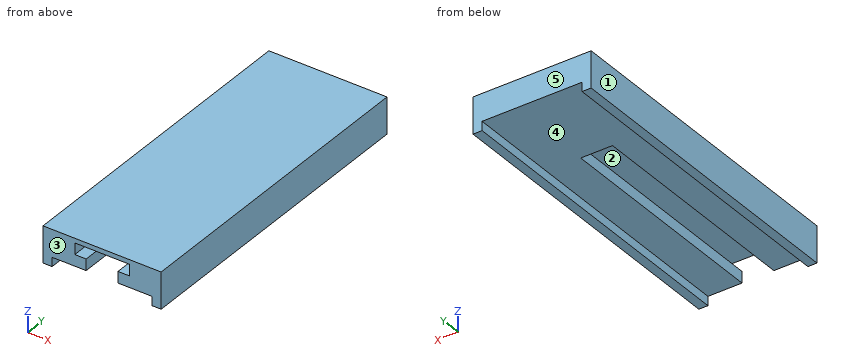
```python
from build123d import *

# Parameters (mm, degrees)
F1_DEPTH = 70
F3_DEPTH = 50


with BuildPart() as f1:
    # F0 (on Front) → F1 (new body)
    with BuildSketch(Plane.XZ):
        Polygon((-11, -6), (11, -6), (11, -8), (13, -8), (13, 0), (-13, 0), (-13, -8), (-11, -8), align=None)
    extrude(amount=-F1_DEPTH)

    # F2 (on face) → F3 (cut)
    with BuildSketch(Plane.XZ):
        Polygon((-3.5, -3.5), (-3.5, -6), (3.5, -6), (3.5, -3.5), (6, -3.5), (6, -1), (-6, -1), (-6, -3.5), align=None)
    extrude(amount=-F3_DEPTH, mode=Mode.SUBTRACT)


solid = f1.part
```
Work out the finished part from the listing and answer in its coordinate system (mm). Face numbers are marked on the shaded views. A direction names the side the tool comes from. Round coordinates to 2 decimals unless told otherwise and drop trailing zeros. Write each loop counter-clockwise with the first axis right and the second up, starting at its lowest first coordinate (ties: lowest second). Pieces come first, ordered by that corner, then holes.
1) A cutting plane is placed at D-D on y = 33. Determine the outline of the cut face in (x, z), and give its area (4 significant figures).
2) Determine the mould class of the marked faces 1, 2 and 3 for opening direction X: pulls with the +X half, pulls with the -X half, needs draft (parallel to the pull), parting line crosses it, or undercut.
3) Which of the six approach directions +Z, -Z, +X, -X, +Y, -Y give full straight-line access (tool end or side, diameter ignored) to the marked faces 4 and 5?
4) A cutting plane is placed at B-B on y = 60. Determine the outline of the cut face in (x, z).
5) A cutting plane is placed at A-A on z = -2.75. Determine the outline of the cut face in (x, y).
6) Consider probe 1 along Z at (x, y) = (4.25, 24); probe 2 along X at (y, z) = (26, -4.5); probe 3 along Z at (x, y) = (8, 48.5). Determine where each line is inside the solid, lowest interval first.
7) Flat-ended cylindrical pins translate along their axes: P1, Ø1.5, axis at x = 1.5, z = -2.5, coming from the -Y side; P2, Ø6, axis at x = 1, y = 18.5, coming from the -Z side. Find the tip coordinate at first contact, or state that the pin passes through.
8) A cutting plane is placed at C-C on x = 1.5. Determine the outline of the cut face in (y, z), and give its area (3 significant figures).
Entries:
1. outline: (-13, -8) - (-11, -8) - (-11, -6) - (-3.5, -6) - (-3.5, -3.5) - (-6, -3.5) - (-6, -1) - (6, -1) - (6, -3.5) - (3.5, -3.5) - (3.5, -6) - (11, -6) - (11, -8) - (13, -8) - (13, 0) - (-13, 0) - close
1. area: 116.5 mm2
2. face 1: pulls with the -X half
2. face 2: undercut
2. face 3: needs draft
3. face 4: -Z, +Y, -Y
3. face 5: +Z, -Z, +X, -X, +Y
4. outline: (-13, -8) - (-11, -8) - (-11, -6) - (11, -6) - (11, -8) - (13, -8) - (13, 0) - (-13, 0) - close
5. outline: (-13, 0) - (-6, 0) - (-6, 50) - (6, 50) - (6, 0) - (13, 0) - (13, 70) - (-13, 70) - close
6. probe 1: z = -6 to -3.5, -1 to 0
6. probe 2: x = -13 to -3.5, 3.5 to 13
6. probe 3: z = -6 to 0
7. P1: stops at y = 50
7. P2: stops at z = -6
8. outline: (0, -1) - (50, -1) - (50, -6) - (70, -6) - (70, 0) - (0, 0) - close
8. area: 170 mm2
